Can you work these out from the drawing? Everything is in mm from the part's minimum corner. Give positions to 0.01 mm unless a question says otherwise; leave off trailing zeros. Write each loop counter-clockwise with the first axis right and the second up, starting at its lowest first coordinate (ties: lowest second). Pieces come first, ordered by that corner, then holes. Notation, with made-up numbers: (-11.75, -7) - (-4.75, -7) arc R19 ccw to (-4.75, 1) - close; hole circle Ø4 at (82, -4.5). An arc over 180 degrees is marked (long way). Use a Markdown table: item, result. Add a question column.
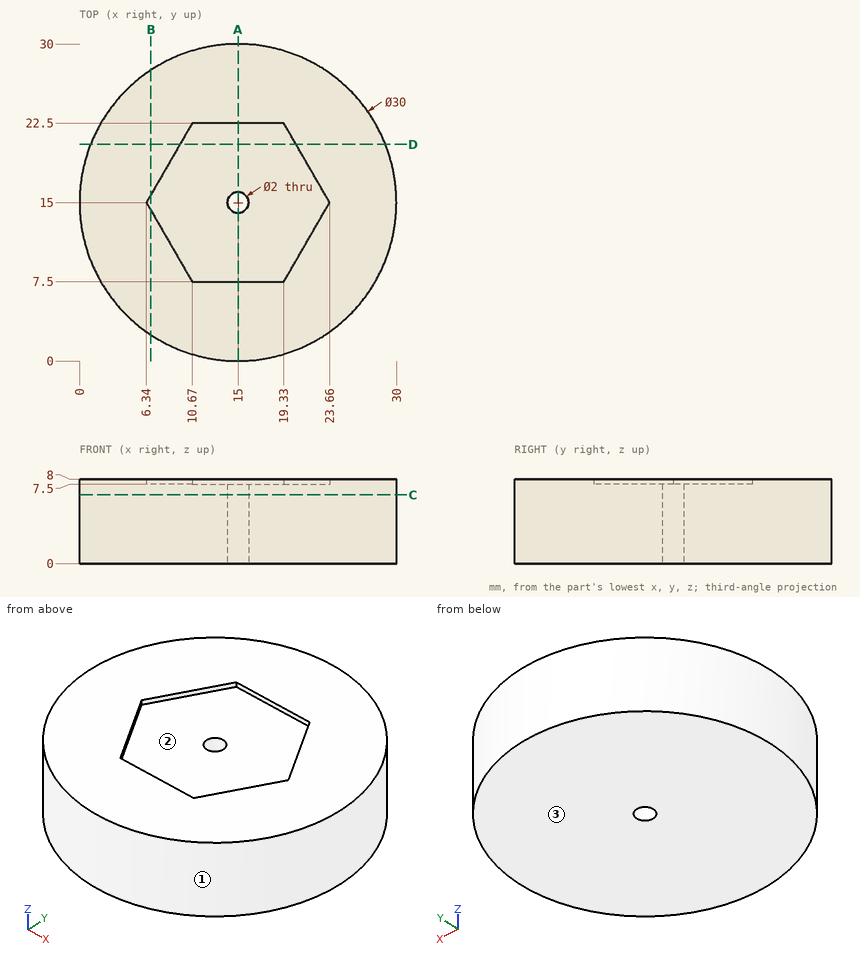
Q1. Suppose I cut it at C-C (z = 6.5). Please give me the cut outline in (x, y), and give its area (3 significant figures).
Q2. Suppose I cut it at B-B (x = 6.75). Please give me the cut outline in (y, z).
Q3. If I drill on probe 1 along Y at (x, z) = (15, 2.25); probe 2 along X at (y, z) = (15.75, 2); probe 3 along X at (y, z) = (26.25, 6.75), over which ranges is the centre line in solid material (lowest first)? Write a range as [from, to].
Q4. Suppose I cut it at D-D (y = 20.5). Please give me the cut outline in (x, z) (1 decimal).
Q5. I'm going to push flat-ended pins straight in: P1, Ø1, axis at x = 21.5, z = 3, coming from the -Y side; P2, Ø4.5, axis at x = 13.5, y = 12.5, coming from the +Z side; P3, Ø1.5, axis at y = 24, z = 5, coming from the +X side. Where does each tip first touch, or does it pass through?
Q6. If we mould it in two halves opening along Y, with no side actions, what happens to the marked faces 1, 2 and 3? For each: released by +Y, released by -Y, zero draft, split by the parting line, or undercut.
Q7. Suppose I cut it at A-A (x = 15). Please give me the cut outline in (y, z).
Derived:
| question | item | result |
|---|---|---|
| 1 | outline | circle Ø30 at (15, 15); hole circle Ø2 at (15, 15) |
| 1 | area | 704 mm² |
| 2 | outline | (2.47, 0) - (27.53, 0) - (27.53, 8) - (15.71, 8) - (15.71, 7.5) - (14.29, 7.5) - (14.29, 8) - (2.47, 8) - close |
| 3 | probe 1 | [0, 14], [16, 30] |
| 3 | probe 2 | [0.02, 14.34], [15.66, 29.98] |
| 3 | probe 3 | [5.08, 24.92] |
| 4 | outline | (1, 0) - (29, 0) - (29, 8) - (20.5, 8) - (20.5, 7.5) - (9.5, 7.5) - (9.5, 8) - (1, 8) - close |
| 5 | P1 | y = 1.25 |
| 5 | P2 | z = 7.5 |
| 5 | P3 | x = 27.53 |
| 6 | face 1 | split by the parting line |
| 6 | face 2 | undercut |
| 6 | face 3 | zero draft |
| 7 | outline | (0, 0) - (14, 0) - (14, 7.5) - (7.5, 7.5) - (7.5, 8) - (0, 8) - close; (16, 0) - (30, 0) - (30, 8) - (22.5, 8) - (22.5, 7.5) - (16, 7.5) - close |
